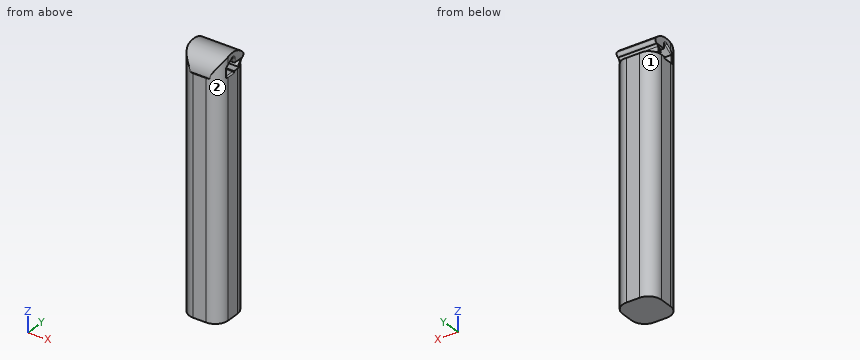
from build123d import *

# Parameters (mm, degrees)
F0_W         = 15
F0_H         = 90
F1_DEPTH     = 15
F3_DEPTH     = 7.5
F4_DEPTH     = 7.5
F5_F1_R      = 0.5
F5_F2_R      = 0.5
F6_R         = 0.5
F7_T1_DEPTH  = 24.4510456068
F8_T1_DEPTH  = 115
F8_T6_DEPTH  = 115
F8_T11_DEPTH = 115


# Not quite as in the source:
# - a fillet or chamfer that OpenCascade refuses, or shapes differently, is made with other operations: its cross-section is extruded or revolved along the edge and cut away or added


with BuildPart() as f1:
    # F0 (on Front) → F1 (new body)
    with BuildSketch(Plane.XZ):
        Rectangle(F0_W, F0_H)
    extrude(amount=F1_DEPTH)

    # F2 (on Right) → F3 (join, symmetric)
    with BuildSketch(Plane.YZ):
        with BuildLine():
            Line((-2.532008104, 48.1942993341), (-0.9043752619, 48.1942993341))
            ThreePointArc((-0.9043752619, 48.1942993341), (-14.6602935003, 43.7750522985), (-0.289426955, 45.269450398))
            Line((-0.289426955, 45.269450398), (-6.7935246953, 45.269450398))
            Line((-6.7935246953, 45.269450398), (-6.7935246953, 43.9416393638))
            Line((-6.7935246953, 43.9416393638), (-10.9625607729, 43.9416393638))
            Line((-10.9625607729, 43.9416393638), (-10.9625607729, 48.1942993341))
            Line((-10.9625607729, 48.1942993341), (-6.7935246953, 50.9531982243))
            Line((-6.7935246953, 50.9531982243), (-6.7935246953, 48.1942993341))
            Line((-6.7935246953, 48.1942993341), (-2.9029950965, 48.1942993341))
            Line((-2.9029950965, 48.1942993341), (-2.532008104, 48.1942993341))
        make_face()
    extrude(amount=F3_DEPTH, both=True)

    # F2 (on Right) → F4 (join, symmetric)
    with BuildSketch(Plane.YZ):
        Polygon((-3.1812353409, 47.4117453826), (-2.9029950965, 48.1942993341), (-4.7579342499, 45.9584258497), (-3.6979690194, 45.9584258497), align=None)
        Polygon((-3.1812353409, 47.4117453826), (-2.532008104, 48.1942993341), (-2.9029950965, 48.1942993341), align=None)
    extrude(amount=F4_DEPTH, both=True)

    # F5: fillet of radius 0.5 on 7 edges, made by hand

    # F5_f1
    f5_f1_edges = [f1.edges().sort_by_distance(p)[0] for p in [
        (0, -6.7935246953, 50.9531982243),
    ]]
    fillet(f5_f1_edges, radius=F5_F1_R)

    # F5_f2
    f5_f2_edges = [f1.edges().sort_by_distance(p)[0] for p in [
        (7.5, -9.2660086927, 49.3170086521),
        (7.5, -10.9625607729, 46.597149667),
        (7.5, -8.8780427341, 45),
        (-7.5, -6.7935246953, 49.1085250933),
        (0, -6.7935246953, 48.1942993341),
        (7.5, -6.7935246953, 49.1085250933),
        (7.5, -7.0568455439, 50.4631858413),
        (-7.5, -7.0568455439, 50.4631858413),
    ]]
    fillet(f5_f2_edges, radius=F5_F2_R)

    # F6
    f6_edges = [f1.edges().sort_by_distance(p)[0] for p in [
        (-7.5, -8.878043, 45),
        (-7.5, -10.962561, 46.59715),
    ]]
    fillet(f6_edges, radius=F6_R)

    # F7: fillet of radius 1 on 1 edges, made by hand

    # F7_s2 → F7_t1 (cut)
    with BuildSketch(Plane.YZ.offset(-12.2255228034)):
        with BuildLine():
            ThreePointArc((-1.8842228199, 49.8107118079), (-1.7364138721, 48.8134688286), (-2.532008104, 48.1942993341))
            Line((-2.532008104, 48.1942993341), (-0.9043752619, 48.1942993341))
            ThreePointArc((-0.9043752619, 48.1942993341), (-1.3414912221, 49.0345169623), (-1.8842228199, 49.8107118079))
        make_face()
    extrude(amount=F7_T1_DEPTH, mode=Mode.SUBTRACT)

    # F8: fillet of radius 5 on 4 edges, made by hand

    # F8_s2 → F8_t1 (cut)
    with BuildSketch(Plane.XY.offset(-57.5)):
        with BuildLine():
            ThreePointArc((-7.5, -10), (-6.0355339059, -13.5355339059), (-2.5, -15))
            Line((-2.5, -15), (-7.5, -15))
            Line((-7.5, -15), (-7.5, -10))
        make_face()
        with BuildLine():
            ThreePointArc((7.5, -10), (6.0355339059, -13.5355339059), (2.5, -15))
            Line((2.5, -15), (7.5, -15))
            Line((7.5, -15), (7.5, -10))
        make_face()
    extrude(amount=F8_T1_DEPTH, mode=Mode.SUBTRACT)


with BuildPart() as f8_tool4:
    # F8_s5 → F8_t6 (new body)
    with BuildSketch(Plane.XY.offset(57.5)):
        with BuildLine():
            ThreePointArc((-7.5, -5), (-6.0355339059, -1.4644660941), (-2.5, 0))
            Line((-2.5, 0), (-7.5, 0))
            Line((-7.5, 0), (-7.5, -5))
        make_face()
    extrude(amount=-F8_T6_DEPTH)

    split(bisect_by=Plane.XY.offset(45.269450398), keep=Keep.BOTTOM)


with BuildPart() as f1_1:
    add(f1.part)

    # F8_t3: cut F8_tool4
    add(f8_tool4.part, mode=Mode.SUBTRACT)


with BuildPart() as f8_tool9:
    # F8_s10 → F8_t11 (new body)
    with BuildSketch(Plane.XY.offset(-57.5)):
        with BuildLine():
            ThreePointArc((7.5, -5), (6.0355339059, -1.4644660941), (2.5, 0))
            Line((2.5, 0), (7.5, 0))
            Line((7.5, 0), (7.5, -5))
        make_face()
    extrude(amount=F8_T11_DEPTH)

    split(bisect_by=Plane.XY.offset(45.269450398), keep=Keep.BOTTOM)


with BuildPart() as f1_2:
    add(f1_1.part)

    # F8_t8: cut F8_tool9
    add(f8_tool9.part, mode=Mode.SUBTRACT)


solid = f1_2.part
Work out the finished part from the listing and answer in its coordinate system (mm). Face numbers are marked on the shaded views. A direction names the side the tool comes from. Coordinates: 2 decimals unless noted, no trailing zeros. Loops run counter-clockwise (first coordinate to the right, second up) from the corner with the lowest first, then second, coordinate; pieces in that order, holes last. Notation, with made-up numbers: (89, -25.5) -> (123, -25.5) arc R17 ccw to (123, -21.5) -> close; hole circle Ø1 at (-35.75, -28). An arc over 180 degrees is marked (long way). Write each question's results on one line, items separated by ' | '. Start each with the question number.
1) Find section A-A on z = 13. Determine the outline of the cut face in (x, y).
2) Flat-ended cylindrical pins translate along their axes: P1, Ø8, axis at x = 1.5, y = -3, coming from the +Z side; P2, Ø1.6, axis at x = -3, z = 46, coming from the +Y side; P3, Ø0.7, axis at x = 0, z = 49, coming from the -Y side; P4, Ø8, axis at x = 2.5, z = 4, coming from the +Y side. Find the tip coordinate at first contact, or state that the pin passes through.
3) Consider line 1 along Z through (x, y) = (-3.25, -3.75); line 2 along Z through (x, y) = (0.75, -4.5); line 3 along X through (y, z) = (-4.75, -4). Determine where each line is inside the solid, lowest interval first.
4) Find section C-C on y = -13.5. Determine the outline of the cut face in (x, z).
5) Find section B-B on x = -0.5. Determine the outline of the cut face in (y, z), then the cut area to 3 significant figures.
6) For the marked faces 1 and 2, determine the directions among +Z, -Z, +X, -X, +Y, -Y from which every point of the face is accessible in a straight line to the end or side of a thin tool.
Response values:
1) outline: (-7.5, -10) arc R5 ccw to (-2.5, -15) -> (2.5, -15) arc R5 ccw to (7.5, -10) -> (7.5, -5) arc R5 ccw to (2.5, 0) -> (-2.5, 0) arc R5 ccw to (-7.5, -5) -> close
2) P1: stops at z = 52.51 | P2: stops at y = -0.29 | P3: stops at y = -13.98 | P4: stops at y = 0
3) line 1: z = -45 to 45.27, 45.96 to 47.17, 48.19 to 51.46 | line 2: z = -45 to 45.27, 45.96 to 46.27, 48.19 to 51.86 | line 3: x = -7.49 to 7.49
4) outline: (-6.07, -45) -> (6.07, -45) -> (6.07, 49.44) -> (-6.07, 49.44) -> close
5) outline: (-15, -45) -> (0, -45) -> (0, 45) -> (-0.29, 45) arc R7.26 ccw to (-0.29, 45.27) -> (-6.79, 45.27) -> (-6.79, 45) -> (-10.96, 45) -> (-10.96, 48.19) -> (-7.57, 50.44) arc R0.5 cw to (-6.79, 50.02) -> (-6.79, 48.69) arc R0.5 ccw to (-6.29, 48.19) -> (-2.9, 48.19) -> (-4.76, 45.96) -> (-3.7, 45.96) -> (-3.18, 47.41) -> (-2.53, 48.19) arc R1 ccw to (-1.88, 49.81) arc R7.26 ccw to (-14.81, 45) -> (-15, 45) -> close | area: 1,400 mm^2
6) face 1: -Z, -X, +Y | face 2: +Z, -Z, +X, -Y
